Could you check a few things on this drawing? It's one solid part, dimensions in mm from its lowest x, y, z. A direction names the side the tool comes from. Give positions to 0.01 mm unless a question says otherwise; leave off trailing zeros. Order: outer loops, then holes, each group sorted by start corner. A loop starts at its lowest first (then second) coordinate and runs counter-clockwise, first axis right, second up.
(1) Imagine slicing it at A-A, the plane y = 11.5. Write out the boundary of the cut face in (x, z), then the cut area to 3 significant figures.
(2) Imagine slicing it at B-B, the plane z = 11. Write out the boundary of the cut face in (x, y).
(3) If we mould it in two halves opening along Z, with no side actions, what happens to the marked faces 1, 2 and 3? For each: released by +Z, released by -Z, zero draft, split by the parting line, or undercut.
(4) Imagine slicing it at C-C, the plane x = 12. Write out the boundary of the cut face in (y, z), then the cut area to 3 significant figures.
(5) Imagine slicing it at D-D, the plane z = 4. Write out the boundary of the cut face in (x, y), then the cut area to 3 significant figures.
(6) Will these pins go through, and if not, where does the flat tip stop? pin 1 (3 mm diameter, centred on y = 6.5, z = 13, fed in from -X); pin 2 (4 mm diameter, centred on x = 11, y = 5, fed in from -Z); pin 3 (4.5 mm diameter, centred on x = 3, z = 11, fed in from -Y).
(7) If I drill on probe 1 along X at (y, z) = (12.3, 11); probe 2 along Y at (x, z) = (11, 14.8); probe 3 along X at (y, z) = (4.75, 11), over which ranges is the centre line in solid material (lowest first)?
(8) On a 3-axis mill with a long thin cutter (end or side, diameter ignored), from which of +Z, -Z, +X, -X, +Y, -Y can I reach the whole of each face in a straight line? I mean the marked faces 4 and 5. Say none if no direction works.
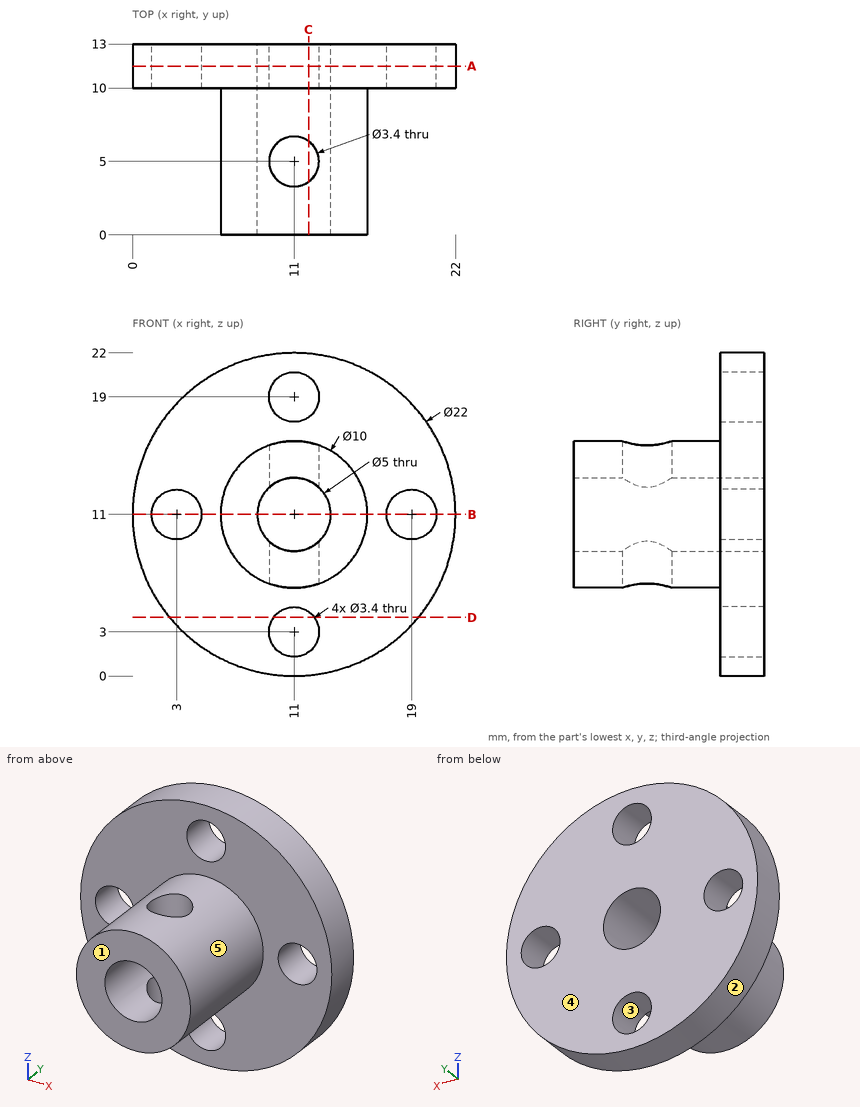
Answer block:
1. outline: circle Ø22 at (11, 11); hole circle Ø3.4 at (3, 11); hole circle Ø5 at (11, 11); hole circle Ø3.4 at (11, 3); hole circle Ø3.4 at (11, 19); hole circle Ø3.4 at (19, 11)
1. area: 324 mm2
2. outline: (0, 10) - (1.3, 10) - (1.3, 13) - (0, 13) - close; (4.7, 10) - (6, 10) - (6, 0) - (8.5, 0) - (8.5, 13) - (4.7, 13) - close; (13.5, 0) - (16, 0) - (16, 10) - (17.3, 10) - (17.3, 13) - (13.5, 13) - close; (20.7, 10) - (22, 10) - (22, 13) - (20.7, 13) - close
3. face 1: zero draft
3. face 2: split by the parting line
3. face 3: undercut
4. outline: (0, 6.1) - (3.63, 6.1) - (3.63, 8.71) - (0, 8.71) - close; (0, 13.29) - (3.63, 13.29) - (3.63, 15.9) - (0, 15.9) - close; (6.37, 6.1) - (10, 6.1) - (10, 4.37) - (13, 4.37) - (13, 8.71) - (6.37, 8.71) - close; (6.37, 13.29) - (13, 13.29) - (13, 17.63) - (10, 17.63) - (10, 15.9) - (6.37, 15.9) - close; (10, 0.05) - (13, 0.05) - (13, 1.63) - (10, 1.63) - close; (10, 20.37) - (13, 20.37) - (13, 21.95) - (10, 21.95) - close
4. area: 73.3 mm2
5. outline: (2.51, 10) - (9.63, 10) - (9.63, 13) - (2.51, 13) - close; (12.37, 10) - (19.49, 10) - (19.49, 13) - (12.37, 13) - close
5. area: 42.7 mm2
6. pin 1: stops at x = 6.03
6. pin 2: stops at z = 6
6. pin 3: stops at y = 10
7. probe 1: x = 0 to 1.3, 4.7 to 8.5, 13.5 to 17.3, 20.7 to 22
7. probe 2: y = 0 to 3.3, 6.7 to 13
7. probe 3: x = 6 to 8.5, 13.5 to 16
8. face 4: +Z, -Z, +X, -X, +Y
8. face 5: -Y
